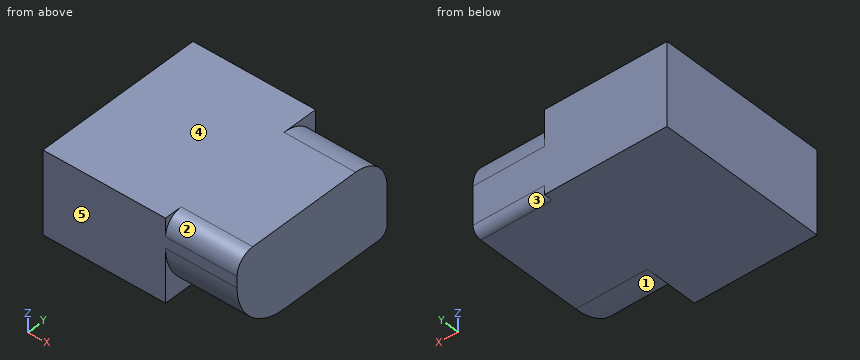
from build123d import *

# Parameters (mm, degrees)
F0_W     = 43.5045808554
F0_H     = 29.3690226972
F1_DEPTH = 60.706
F3_DEPTH = 25.4


with BuildPart() as f1:
    # F0 (on Front) → F1 (new body)
    with BuildSketch(Plane.XZ):
        with Locations((21.7522904277, -14.6845113486)):
            Rectangle(F0_W, F0_H)
    extrude(amount=F1_DEPTH)

    # F2 (on face) → F3 (join)
    with BuildSketch(Plane.YZ.offset(43.5045808554)):
        with BuildLine():
            ThreePointArc((-3.175, -29.3690226972), (-0.9299359697, -28.4390867275), (0, -26.1940226972))
            Line((0, -26.1940226972), (0, -12.7))
            ThreePointArc((0, -12.7), (-3.7197438789, -3.7197438789), (-12.7, 0))
            Line((-12.7, 0), (-54.356, 0))
            ThreePointArc((-54.356, 0), (-58.8461280605, -1.8598719395), (-60.706, -6.35))
            Line((-60.706, -6.35), (-60.706, -10.3190226972))
            ThreePointArc((-60.706, -10.3190226972), (-55.1263841816, -23.7894068788), (-41.656, -29.3690226972))
            Line((-41.656, -29.3690226972), (-3.175, -29.3690226972))
        make_face()
    extrude(amount=F3_DEPTH)


solid = f1.part
Could you check a few things on this model? Use its own coordinates, in mm. Face numbers are marked on the shaded views. A direction names the side the tool comes from. Give positions to 0.01 mm unless a question says otherwise; leave off trailing zeros. Order: outer loops, then holes, each group sorted by start corner. A loop starts at its lowest first (then second) coordinate and runs counter-clockwise, first axis right, second up. Notation, with made-up numbers: (59, 51) - (75, 51) arc R15 ccw to (75, 70) - close; hole circle Ø6 at (29.5, 11). An arc over 180 degrees is marked (long way). One line per question, with ' | ' between items. Start each with the question number.
Item 1: I'm going to push a flat-ended pin straight in: pin 1 Ø3 at (x, y) = (53, -46) entering from -Z. Where does the tip first touch, or does it pass through?
Item 2: I need wall thicknesses on probe 1 along Z at (x, y) = (56, -47.5); probe 2 along Y at (x, z) = (46.5, -3.25); probe 3 along Y at (x, z) = (49, -26). Which ranges of each line are inside material? Lowest first, please. Write a range as [from, to].
Item 3: For the marked faces 1, 2, 3, 4 and 5, which set-ups out of +Z, -Z, +X, -X, +Y, -Y let a thin tool reach every point of the face, with its end or its side?
Item 4: I want a section at A-A on x = 49. Write out the boundary of the cut face in (y, z) (3 decimals), then the cut area to 3 significant figures.
Item 5: I want a section at B-B on z = -4.25. Write out the boundary of the cut face in (x, y).
Item 6: I want a section at C-C on z = -21.5. Write out the boundary of the cut face in (x, y), then the cut area to 3 significant figures.
Verdict:
1) pin 1: z = -29.16
2) probe 1: [-28.45, 0] | probe 2: [-59.9, -4.22] | probe 3: [-52.47, 0]
3) face 1: -Z, +X, -Y | face 2: +Z, +X, -Y | face 3: -Z, +X, +Y | face 4: +Z, +X, -X, +Y, -Y | face 5: +Z, -Z, +X, -X, -Y
4) outline: (-60.706, -10.319) arc R19.05 ccw to (-41.656, -29.369) - (-3.175, -29.369) arc R3.175 ccw to (0, -26.194) - (0, -12.7) arc R12.7 ccw to (-12.7, 0) - (-54.356, 0) arc R6.35 ccw to (-60.706, -6.35) - close | area: 1,660 mm^2
5) outline: (0, -60.71) - (43.5, -60.71) - (43.5, -60.35) - (68.9, -60.35) - (68.9, -3.22) - (43.5, -3.22) - (43.5, 0) - (0, 0) - close
6) outline: (0, -60.71) - (43.5, -60.71) - (43.5, -57.08) - (68.9, -57.08) - (68.9, 0) - (0, 0) - close | area: 4,090 mm^2
